```python
from build123d import *
from build123d.topology import SkipClean

# Parameters (mm, degrees)
SKETCH1_R           = 2.5
BOSS_EXTRUDE1_DEPTH = 10
SKETCH2_R           = 2.5
BOSS_EXTRUDE2_DEPTH = 10
SKETCH3_R           = 5
SKETCH3_R_2         = 2.5
BOSS_EXTRUDE3_DEPTH = 6
SKETCH4_R           = 2.5
CUT_EXTRUDE1_DEPTH  = 41.209967862
CUT_EXTRUDE2_DEPTH  = 41.209967862


with BuildPart() as part:
    # Sketch1 → Boss-Extrude1 (new body)
    with BuildSketch(Plane(origin=(4.043870029, 0, 0), x_dir=(0, 0, -1), z_dir=(1, 0, 0))):
        with BuildLine():
            ThreePointArc((-10.029541992, 0.342879069), (-9.019080639, -0.304016541), (-7.862233613, -0.622153359))
            ThreePointArc((-7.862233613, -0.622153359), (-7.876528296, -1.122077366), (-7.862233613, -1.622001374))
            ThreePointArc((-7.862233613, -1.622001374), (-9.019080639, -1.940138191), (-10.029541992, -2.587033801))
            ThreePointArc((-10.029541992, -2.587033801), (-9.992100042, -2.842856482), (-9.948655897, -3.097728508))
            ThreePointArc((-9.948655897, -3.097728508), (-8.787748306, -3.400713063), (-7.58921172, -3.345793765))
            ThreePointArc((-7.58921172, -3.345793765), (-7.448321757, -3.82566705), (-7.280241692, -4.296705735))
            ThreePointArc((-7.280241692, -4.296705735), (-8.282158911, -4.956757219), (-9.043263028, -5.884241235))
            ThreePointArc((-9.043263028, -5.884241235), (-8.928600062, -6.115972863), (-8.808522437, -6.344945585))
            ThreePointArc((-8.808522437, -6.344945585), (-7.610806331, -6.274360846), (-6.487901298, -5.851761317))
            ThreePointArc((-6.487901298, -5.851761317), (-6.20561798, -6.264610538), (-5.90020538, -6.660655353))
            ThreePointArc((-5.90020538, -6.660655353), (-6.649118154, -7.598011066), (-7.086362862, -8.715294889))
            ThreePointArc((-7.086362862, -8.715294889), (-6.905702889, -8.900251959), (-6.720745819, -9.080911932))
            ThreePointArc((-6.720745819, -9.080911932), (-5.603461996, -8.643667224), (-4.666106283, -7.89475445))
            ThreePointArc((-4.666106283, -7.89475445), (-4.270061468, -8.20016705), (-3.857212247, -8.482450368))
            ThreePointArc((-3.857212247, -8.482450368), (-4.279811776, -9.605355401), (-4.350396515, -10.803071507))
            ThreePointArc((-4.350396515, -10.803071507), (-4.121423793, -10.923149132), (-3.889692165, -11.037812099))
            ThreePointArc((-3.889692165, -11.037812099), (-2.962208149, -10.276707981), (-2.302156665, -9.274790762))
            ThreePointArc((-2.302156665, -9.274790762), (-1.83111798, -9.442870827), (-1.351244695, -9.583760791))
            ThreePointArc((-1.351244695, -9.583760791), (-1.406163992, -10.782297376), (-1.103179437, -11.943204968))
            ThreePointArc((-1.103179437, -11.943204968), (-0.848307411, -11.986649113), (-0.592484731, -12.024091063))
            ThreePointArc((-0.592484731, -12.024091063), (0.054410879, -11.01362971), (0.372547697, -9.856782684))
            ThreePointArc((0.372547697, -9.856782684), (0.872471704, -9.871077366), (1.372395712, -9.856782684))
            ThreePointArc((1.372395712, -9.856782684), (1.690532529, -11.01362971), (2.337428139, -12.024091063))
            ThreePointArc((2.337428139, -12.024091063), (2.59325082, -11.986649113), (2.848122846, -11.943204968))
            ThreePointArc((2.848122846, -11.943204968), (3.151107401, -10.782297376), (3.096188103, -9.583760791))
            ThreePointArc((3.096188103, -9.583760791), (3.576061388, -9.442870827), (4.047100073, -9.274790762))
            ThreePointArc((4.047100073, -9.274790762), (4.707151558, -10.276707981), (5.634635573, -11.037812099))
            ThreePointArc((5.634635573, -11.037812099), (5.866367201, -10.923149132), (6.095339923, -10.803071507))
            ThreePointArc((6.095339923, -10.803071507), (6.024755184, -9.605355401), (5.602155655, -8.482450368))
            ThreePointArc((5.602155655, -8.482450368), (6.015004877, -8.20016705), (6.411049691, -7.89475445))
            ThreePointArc((6.411049691, -7.89475445), (7.348405404, -8.643667224), (8.465689227, -9.080911932))
            ThreePointArc((8.465689227, -9.080911932), (8.650646297, -8.900251959), (8.83130627, -8.715294889))
            ThreePointArc((8.83130627, -8.715294889), (8.394061563, -7.598011066), (7.645148788, -6.660655353))
            ThreePointArc((7.645148788, -6.660655353), (7.950561388, -6.264610538), (8.232844706, -5.851761317))
            ThreePointArc((8.232844706, -5.851761317), (9.355749739, -6.274360846), (10.553465846, -6.344945585))
            ThreePointArc((10.553465846, -6.344945585), (10.67354347, -6.115972863), (10.788206437, -5.884241235))
            ThreePointArc((10.788206437, -5.884241235), (10.02710232, -4.956757219), (9.0251851, -4.296705735))
            ThreePointArc((9.0251851, -4.296705735), (9.193265165, -3.82566705), (9.334155129, -3.345793765))
            ThreePointArc((9.334155129, -3.345793765), (10.532691714, -3.400713063), (11.693599306, -3.097728508))
            ThreePointArc((11.693599306, -3.097728508), (11.737043451, -2.842856482), (11.774485401, -2.587033801))
            ThreePointArc((11.774485401, -2.587033801), (10.764024048, -1.940138191), (9.607177022, -1.622001374))
            ThreePointArc((9.607177022, -1.622001374), (9.621471704, -1.122077366), (9.607177022, -0.622153359))
            ThreePointArc((9.607177022, -0.622153359), (10.764024048, -0.304016541), (11.774485401, 0.342879069))
            ThreePointArc((11.774485401, 0.342879069), (11.737043451, 0.598701749), (11.693599306, 0.853573775))
            ThreePointArc((11.693599306, 0.853573775), (10.532691714, 1.156558331), (9.334155129, 1.101639033))
            ThreePointArc((9.334155129, 1.101639033), (9.193265165, 1.581512318), (9.0251851, 2.052551003))
            ThreePointArc((9.0251851, 2.052551003), (10.02710232, 2.712602487), (10.788206437, 3.640086503))
            ThreePointArc((10.788206437, 3.640086503), (10.67354347, 3.871818131), (10.553465846, 4.100790853))
            ThreePointArc((10.553465846, 4.100790853), (9.355749739, 4.030206114), (8.232844706, 3.607606585))
            ThreePointArc((8.232844706, 3.607606585), (7.950561388, 4.020455806), (7.645148788, 4.416500621))
            ThreePointArc((7.645148788, 4.416500621), (8.394061563, 5.353856334), (8.83130627, 6.471140157))
            ThreePointArc((8.83130627, 6.471140157), (8.650646297, 6.656097227), (8.465689227, 6.8367572))
            ThreePointArc((8.465689227, 6.8367572), (7.348405404, 6.399512492), (6.411049691, 5.650599718))
            ThreePointArc((6.411049691, 5.650599718), (6.015004877, 5.956012318), (5.602155655, 6.238295636))
            ThreePointArc((5.602155655, 6.238295636), (6.024755184, 7.361200669), (6.095339923, 8.558916775))
            ThreePointArc((6.095339923, 8.558916775), (5.866367201, 8.6789944), (5.634635573, 8.793657366))
            ThreePointArc((5.634635573, 8.793657366), (4.707151558, 8.032553249), (4.047100073, 7.03063603))
            ThreePointArc((4.047100073, 7.03063603), (3.576061388, 7.198716095), (3.096188103, 7.339606058))
            ThreePointArc((3.096188103, 7.339606058), (3.151107401, 8.538142644), (2.848122846, 9.699050235))
            ThreePointArc((2.848122846, 9.699050235), (2.59325082, 9.74249438), (2.337428139, 9.779936331))
            ThreePointArc((2.337428139, 9.779936331), (1.690532529, 8.769474978), (1.372395712, 7.612627952))
            ThreePointArc((1.372395712, 7.612627952), (0.872471704, 7.626922634), (0.372547697, 7.612627952))
            ThreePointArc((0.372547697, 7.612627952), (0.054410879, 8.769474978), (-0.592484731, 9.779936331))
            ThreePointArc((-0.592484731, 9.779936331), (-0.848307411, 9.74249438), (-1.103179437, 9.699050235))
            ThreePointArc((-1.103179437, 9.699050235), (-1.406163992, 8.538142644), (-1.351244695, 7.339606058))
            ThreePointArc((-1.351244695, 7.339606058), (-1.83111798, 7.198716095), (-2.302156665, 7.03063603))
            ThreePointArc((-2.302156665, 7.03063603), (-2.962208149, 8.032553249), (-3.889692165, 8.793657366))
            ThreePointArc((-3.889692165, 8.793657366), (-4.121423793, 8.6789944), (-4.350396515, 8.558916775))
            ThreePointArc((-4.350396515, 8.558916775), (-4.279811776, 7.361200669), (-3.857212247, 6.238295636))
            ThreePointArc((-3.857212247, 6.238295636), (-4.270061468, 5.956012318), (-4.666106283, 5.650599718))
            ThreePointArc((-4.666106283, 5.650599718), (-5.603461996, 6.399512492), (-6.720745819, 6.8367572))
            ThreePointArc((-6.720745819, 6.8367572), (-6.905702889, 6.656097227), (-7.086362862, 6.471140157))
            ThreePointArc((-7.086362862, 6.471140157), (-6.649118154, 5.353856334), (-5.90020538, 4.416500621))
            ThreePointArc((-5.90020538, 4.416500621), (-6.20561798, 4.020455806), (-6.487901298, 3.607606585))
            ThreePointArc((-6.487901298, 3.607606585), (-7.610806331, 4.030206114), (-8.808522437, 4.100790853))
            ThreePointArc((-8.808522437, 4.100790853), (-8.928600062, 3.871818131), (-9.043263028, 3.640086503))
            ThreePointArc((-9.043263028, 3.640086503), (-8.282158911, 2.712602487), (-7.280241692, 2.052551003))
            ThreePointArc((-7.280241692, 2.052551003), (-7.448321757, 1.581512318), (-7.58921172, 1.101639033))
            ThreePointArc((-7.58921172, 1.101639033), (-8.787748306, 1.156558331), (-9.948655897, 0.853573775))
            ThreePointArc((-9.948655897, 0.853573775), (-9.992100042, 0.598701749), (-10.029541992, 0.342879069))
        make_face()
        with Locations(Location((0.872471704, -1.122077366, 0), (0, 0, 180))):
            Circle(SKETCH1_R, mode=Mode.SUBTRACT)
    extrude(amount=-BOSS_EXTRUDE1_DEPTH)

    # Sketch2 → Boss-Extrude2 (add)
    with BuildSketch(Plane(origin=(4.043870029, 0, 0), x_dir=(0, 0, -1), z_dir=(1, 0, 0))):
        with BuildLine():
            Line((-2.754400151, 2.319695512), (17.89623712, 24.080926643))
            ThreePointArc((17.89623712, 24.080926643), (24.964881853, 24.266025619), (25.14998083, 17.197380886))
            Line((25.14998083, 17.197380886), (4.499343559, -4.563850245))
            ThreePointArc((4.499343559, -4.563850245), (-2.569301174, -4.748949221), (-2.754400151, 2.319695512))
        make_face()
        with Locations((21.523108975, 20.639153764)):
            Circle(SKETCH2_R, mode=Mode.SUBTRACT)
    extrude(amount=-BOSS_EXTRUDE2_DEPTH)

    # Sketch3 → Boss-Extrude3 (add)
    with BuildSketch(Plane.ZY.offset(5.956129971)):
        with Locations(Location((-21.523108975, 20.639153764, 0), (0, 0, 223.5))):
            Circle(SKETCH3_R)
        with Locations(Location((-21.523108975, 20.639153764, 0), (0, 0, 180))):
            Circle(SKETCH3_R_2, mode=Mode.SUBTRACT)
    extrude(amount=BOSS_EXTRUDE3_DEPTH)

    # Sketch4 → Cut-Extrude1 (cut, through all)
    with BuildSketch(Plane(origin=(4.043870029, 0, 0), x_dir=(0, 0, -1), z_dir=(1, 0, 0))):
        with Locations((0.872471704, -1.122077366)):
            Circle(SKETCH4_R)
    extrude(amount=-CUT_EXTRUDE1_DEPTH, mode=Mode.SUBTRACT)

    # Sketch6 → Cut-Extrude2 (cut, through all)
    with SkipClean():  # the faces are left unmerged after this step: merging them gives an invalid solid
        with BuildSketch(Plane(origin=(4.043870029, 0, 0), x_dir=(0, 0, -1), z_dir=(1, 0, 0))):
            with BuildLine():
                Line((4.579688985, 10.048212881), (2.187631015, 7.527509733))
                ThreePointArc((2.187631015, 7.527509733), (-2.46576826, 6.965020688), (-6.16100093, 4.08131227))
                Line((-6.16100093, 4.08131227), (-8.58915512, 5.877669916))
                ThreePointArc((-8.58915512, 5.877669916), (-2.68093011, 10.098091069), (4.579688985, 10.048212881))
            make_face()
            with BuildLine():
                Line((11.833432695, 3.164667124), (9.441374725, 0.643963976))
                ThreePointArc((9.441374725, 0.643963976), (9.424184018, -2.969566881), (7.948146758, -6.267932352))
                Line((7.948146758, -6.267932352), (10.39087042, -8.044427405))
                ThreePointArc((10.39087042, -8.044427405), (12.54560297, -2.624359175), (11.833432695, 3.164667124))
            make_face()
        extrude(amount=-CUT_EXTRUDE2_DEPTH, mode=Mode.SUBTRACT)


solid = part.part
```
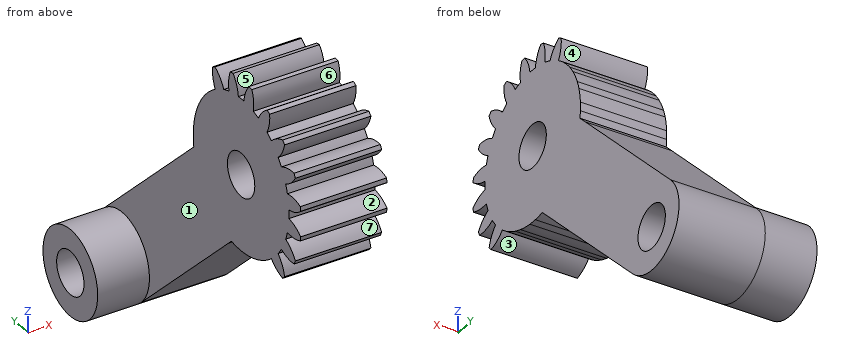
Build history of the part. All positions in model axes, mm. Face numbers are marked on the shaded views. A direction names the side the tool comes from. Round coordinates to 2 decimals unless told otherwise and drop trailing zeros. Loops run counter-clockwise (first coordinate to the right, second up) from the corner with the lowest first, then second, coordinate; pieces in that order, holes last.
Item 1: Saw through at A-A (z = -20). List the corners of the cut face in (x, y), then the cut area to 3 significant figures.
Item 2: Saw through at D-D (y = 5). List the corners of the cut face in (x, z).
Item 3: Two-plate mould, pull along Z, no slides. Class the marked faces 1, 2 and 3: released by +Z, released by -Z, zero draft, split by the parting line, or undercut.
Item 4: Which spindle directions (+Z, -Z, +X, -X, +Y, -Y) get a long thin tool onto all of the face, cutting with end or side? Do the marked faces 4, 5, 6 and 7. Say none if no direction does.
Item 5: Pin check, flat tips, straight feed: P1, Ø6, axis at x = -3, z = -0.5, coming from the +Y side; P2, Ø1.5, axis at x = -10, y = 19.5, coming from the +Z side; P3, Ø6.5, axis at y = -1.12, z = -0.87, coming from the -X side; P4, Ø4, axis at y = 20.64, z = -21.52, coming from the +X side. Stop position of each tip, or through.
Item 6: Saw through at B-B (x = -2). State how many separate pieces and enclosed holes the cut face has, then the cut area to 3 significant figures.
Item 7: Saw through at C-C (z = -5). List the corners of the cut face in (x, y), then the cut area to 3 significant figures.
Item 8: Drill centre lines: line 1 along X through (y, z) = (4.5, -8); line 2 along Y through (x, z) = (-4.75, 6); line 3 along Y through (x, z) = (-5.75, -0.5). Where is each one in solid material? Low to high.
Worked answers:
1. outline: (-11.96, 15.88) - (-5.96, 15.88) - (-5.96, 11.77) - (4.04, 11.77) - (4.04, 18.66) - (-11.96, 18.66) - close; (-11.96, 22.62) - (4.04, 22.62) - (4.04, 25.4) - (-11.96, 25.4) - close
1. area: 130 mm2
2. outline: (-5.96, -13.58) - (4.04, -13.58) - (4.04, 5.38) - (-5.96, 5.38) - close
3. face 1: zero draft
3. face 2: undercut
3. face 3: released by -Z
4. face 4: +X, -X, +Y
4. face 5: +Z, +X, -X
4. face 6: +X, -X
4. face 7: +X, -X, -Y
5. P1: stops at y = 8.91
5. P2: stops at z = -16.54
5. P3: stops at x = -5.96
5. P4: passes through
6. separate pieces: 1
6. enclosed holes: 2
6. area: 489 mm2
7. outline: (-5.96, -10.57) - (4.04, -10.57) - (4.04, 10.49) - (-5.96, 10.49) - close
7. area: 211 mm2
8. line 1: x = -5.96 to 4.04
8. line 2: y = -8.84 to -6.76, -6.54 to 4.29
8. line 3: y = -9.86 to -3.59, 1.35 to 7.62
